Check sheet for the drawn part. Datum: minimum x, y, z corner. Units: mm. A direction names the side the tool comes from. Round coordinates to 2 decimals unless told otherwise and drop trailing zeros. Order: outer loops, then holes, each group sorted by start corner. A loop starts at its lowest first (then second) coordinate and runs counter-clockwise, first axis right, second up. Notation, with made-up numbers: (-17, 43.25) -> (37, 43.25) arc R10 ccw to (37, 48.25) -> close; hole circle Ø1 at (71, 20.5). An arc over 180 degrees is marked (long way). Write item = value, one per line. Start each with the question number.
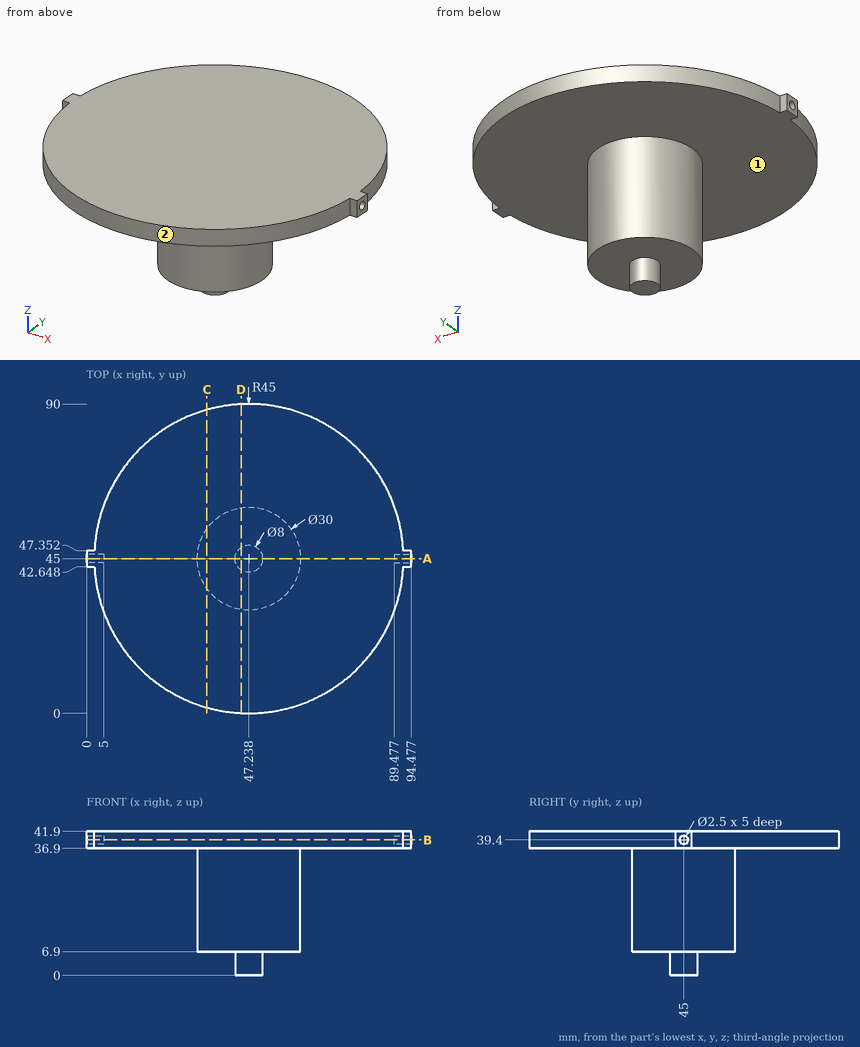
(1) Scan lines: line 1 along X through (y, z) = (29.5, 40) (1 decimal); line 2 along Z through (x, y) = (43, 7); line 3 along Z through (x, y) = (58.5, 36). Record each from-to range of solid material in increasing order. Write a range as from..to.
(2) Cross-section at C-C (x = 35). Enter the section's corners in (y, z).
(3) Cross-section at D-D (x = 45). Enter the section's corners in (y, z) (1 decimal).
(4) Set-up check for the marked faces 1 and 2: record each of +Z, -Z, +X, -X, +Y, -Y from which the full face is reachable in a straight line by a thin tool's end or side.
(5) Cross-section at B-B (z = 39.4). Enter the section's corners in (x, y), and give its area (3 significant figures).
(6) Cross-section at A-A (y = 45). Enter the section's corners in (x, z), and give its area (3 significant figures).
(7) Depth check by flat-ended pin: pin 1 (3 mm diameter, centred on x = 36.5, z = 19.5, fed in from -Y); pin 2 (3 mm diameter, centred on x = 41.5, y = 60, fed in from -Z); pin 3 (2 mm diameter, centred on y = 45, z = 39.4, fed in from +X). Enter the tip coordinate at first touch or a pass-through.
Outcome:
q1.line_1 = 5..89.5
q1.line_2 = 36.9..41.9
q1.line_3 = 6.9..41.9
q2.outline = (1.7, 36.9) -> (36.33, 36.9) -> (36.33, 6.9) -> (53.67, 6.9) -> (53.67, 36.9) -> (88.3, 36.9) -> (88.3, 41.9) -> (1.7, 41.9) -> close
q3.outline = (0.1, 36.9) -> (30.2, 36.9) -> (30.2, 6.9) -> (41.7, 6.9) -> (41.7, 0) -> (48.3, 0) -> (48.3, 6.9) -> (59.8, 6.9) -> (59.8, 36.9) -> (89.9, 36.9) -> (89.9, 41.9) -> (0.1, 41.9) -> close
q4.face_1 = -Z
q4.face_2 = +Z, -Z, -Y
q5.outline = (0, 42.65) -> (2.3, 42.65) arc R45 ccw to (92.18, 42.65) -> (94.48, 42.65) -> (94.48, 43.75) -> (89.48, 43.75) -> (89.48, 46.25) -> (94.48, 46.25) -> (94.48, 47.35) -> (92.18, 47.35) arc R45 ccw to (2.3, 47.35) -> (0, 47.35) -> (0, 46.25) -> (5, 46.25) -> (5, 43.75) -> (0, 43.75) -> close
q5.area = 6,360 mm^2
q6.outline = (0, 36.9) -> (32.24, 36.9) -> (32.24, 6.9) -> (43.24, 6.9) -> (43.24, 0) -> (51.24, 0) -> (51.24, 6.9) -> (62.24, 6.9) -> (62.24, 36.9) -> (94.48, 36.9) -> (94.48, 38.15) -> (89.48, 38.15) -> (89.48, 40.65) -> (94.48, 40.65) -> (94.48, 41.9) -> (0, 41.9) -> (0, 40.65) -> (5, 40.65) -> (5, 38.15) -> (0, 38.15) -> close
q6.area = 1,400 mm^2
q7.pin_1 = 33.18
q7.pin_2 = 6.9
q7.pin_3 = 89.48
